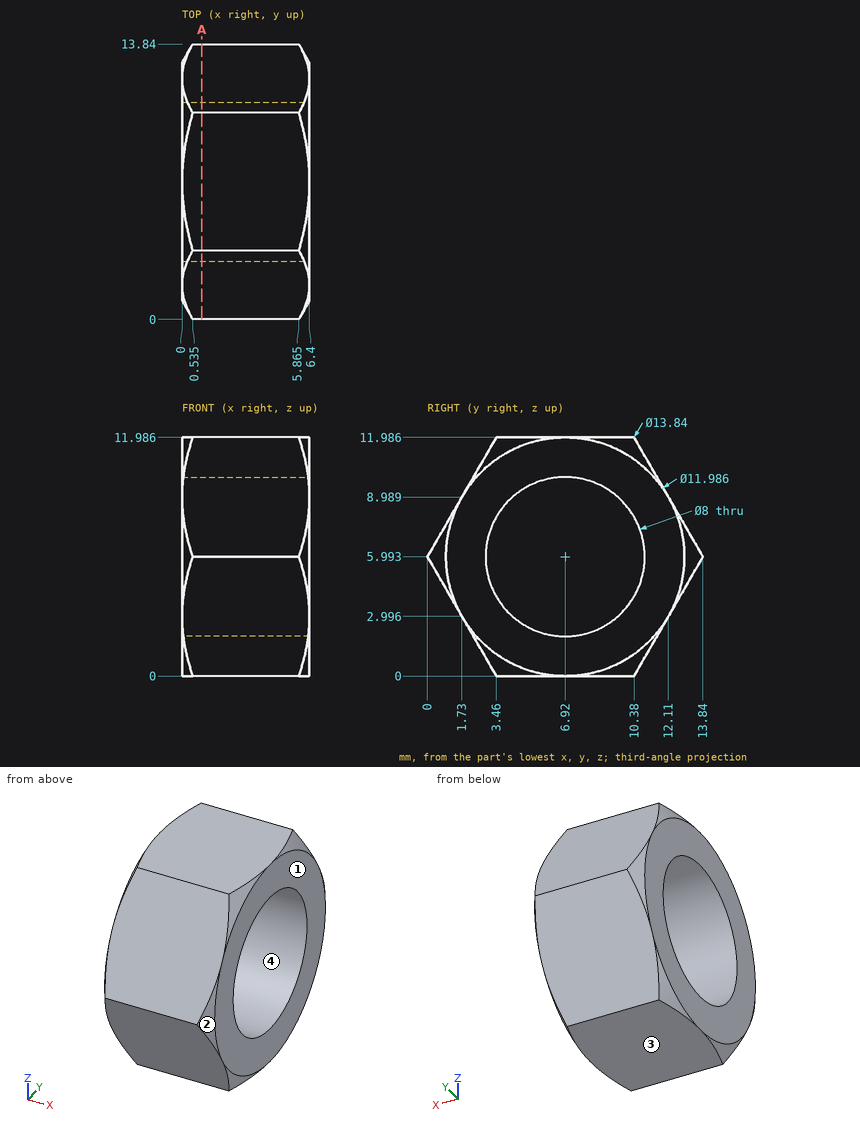
Geometry check sheet. Reference: drawing and pictorial views, mm from the part's lowest x, y, z. Round coordinates to 2 decimals unless told otherwise and drop trailing zeros. Write each loop counter-clockwise with the first axis right and the second up, starting at its lowest first coordinate (ties: lowest second). Pieces come first, ordered by that corner, then holes.
1. Section check A-A on x = 1. Enter the section's corners in (y, z) (1 decimal).
2. Scan lines: L1, parallel to Y at x = 1.25, z = 7.75 (1 decimal); L2, parallel to Z at x = 4.25, y = 10 (1 decimal); L3, parallel to Z at x = 3, y = 9.75 (1 decimal). Record each from-to range of solid material in increasing order.
3. Draft check along Z on the marked faces 1, 2, 3 and 4. Enter one of: +Z half, -Z half, draft (parallel to the pull), parting line (faces both ways), or undercut.
4. Gauge pin test, flat end, axial feed: P1, Ø1, axis at x = 2, y = 1.5, coming from the +Z side (1 decimal). Record the tip position at first contact, or that the pin passes through.
Answer:
1. outline: (0, 6) - (3.5, 0) - (10.4, 0) - (13.8, 6) - (10.4, 12) - (3.5, 12) - close; hole circle Ø8 at (6.9, 6)
2. L1: y = 1 to 3.3, 10.5 to 12.8
2. L2: z = 0 to 3.4, 8.5 to 12
2. L3: z = 0 to 3.2, 8.8 to 12
3. face 1: draft
3. face 2: parting line
3. face 3: -Z half
3. face 4: undercut
4. P1: stops at z = 9.5
